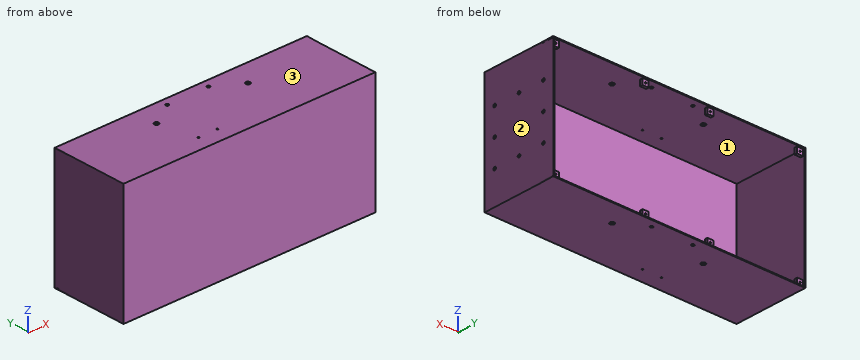
from build123d import *

# Parameters (mm, degrees)
SKETCH1_W            = 855
SKETCH1_H            = 400
BOSS_EXTRUDE1_DEPTH  = 4
SKETCH3_W            = 3
SKETCH3_H            = 394
BOSS_EXTRUDE2_DEPTH  = 200
BOSS_EXTRUDE3_DEPTH  = 3
BOSS_EXTRUDE4_START  = -3
BOSS_EXTRUDE4_DEPTH  = 3
SKETCH10_R           = 5
CUT_EXTRUDE4_DEPTH   = 639.178854241
SKETCH11_R           = 2.5
CUT_EXTRUDE5_DEPTH   = 639.178854241
BOSS_EXTRUDE7_DEPTH  = 3
BOSS_EXTRUDE10_START = -3
BOSS_EXTRUDE10_DEPTH = 3
SKETCH33_W           = 3
SKETCH33_H           = 394
BOSS_EXTRUDE14_DEPTH = 50
SKETCH34_W           = 3
SKETCH34_H           = 394
BOSS_EXTRUDE15_DEPTH = 50
SKETCH36_W           = 20
SKETCH36_H           = 20
BOSS_EXTRUDE16_DEPTH = 9
SKETCH40_R           = 2.5
CUT_EXTRUDE6_DEPTH   = 9
SKETCH44_W           = 20
SKETCH44_H           = 20
BOSS_EXTRUDE18_DEPTH = 9
SKETCH45_R           = 2.5
CUT_EXTRUDE7_DEPTH   = 9
SKETCH46_W           = 20
SKETCH46_H           = 20
BOSS_EXTRUDE19_DEPTH = 9
SKETCH47_R           = 2.5
CUT_EXTRUDE8_DEPTH   = 9
SKETCH48_W           = 20
SKETCH48_H           = 20
BOSS_EXTRUDE20_DEPTH = 9
SKETCH49_R           = 2.5
CUT_EXTRUDE9_DEPTH   = 9
SKETCH50_W           = 20
SKETCH50_H           = 20
BOSS_EXTRUDE21_DEPTH = 9
SKETCH51_R           = 2.5
CUT_EXTRUDE10_DEPTH  = 9
SKETCH52_W           = 20
SKETCH52_H           = 20
BOSS_EXTRUDE22_DEPTH = 9
SKETCH53_R           = 2.5
CUT_EXTRUDE11_DEPTH  = 9
SKETCH58_W           = 20
SKETCH58_H           = 20
BOSS_EXTRUDE25_DEPTH = 9
SKETCH61_R           = 2.5
CUT_EXTRUDE13_DEPTH  = 9
SKETCH62_W           = 20
SKETCH62_H           = 20
BOSS_EXTRUDE26_DEPTH = 9
SKETCH63_R           = 2.5
CUT_EXTRUDE14_DEPTH  = 9
SKETCH64_R           = 7.5
CUT_EXTRUDE15_DEPTH  = 639.906527631
SKETCH65_R           = 5
CUT_EXTRUDE16_DEPTH  = 3


with BuildPart() as part:
    # Sketch1 → Boss-Extrude1 (new body)
    with BuildSketch(Plane(origin=(0, 0, 0), x_dir=(1, 0, 0), z_dir=(0, 1, 0))):
        Rectangle(SKETCH1_W, SKETCH1_H)
    extrude(amount=BOSS_EXTRUDE1_DEPTH)

    # Sketch3 → Boss-Extrude2 (add)
    with BuildSketch(Plane(origin=(0, 4, 0), x_dir=(1, 0, 0), z_dir=(0, 1, 0))):
        Polygon((-424.5, 200), (-424.5, 197), (424.5, 197), (427.5, 197), (427.5, 200), align=None)
        with Locations((426, 0)):
            Rectangle(SKETCH3_W, SKETCH3_H)
        Polygon((-427.5, -197), (-427.5, -200), (427.5, -200), (427.5, -197), (424.5, -197), (-424.5, -197), align=None)
        Polygon((-427.5, 200), (-427.5, -197), (-424.5, -197), (-424.5, 197), (-424.5, 200), align=None)
    extrude(amount=BOSS_EXTRUDE2_DEPTH)

    # Sketch4 → Boss-Extrude3 (add)
    with BuildSketch(Plane.XY.offset(200)):
        with BuildLine():
            ThreePointArc((427.5, 204), (215.207022423, 241.457541713), (0, 254))
            Line((0, 254), (0, 204))
            Line((0, 204), (427.5, 204))
        make_face()
        with BuildLine():
            Line((0, 204), (0, 254))
            ThreePointArc((0, 254), (-215.207022423, 241.457541713), (-427.5, 204))
            Line((-427.5, 204), (0, 204))
        make_face()
        with BuildLine():
            ThreePointArc((427.5, 204), (215.207022423, 241.457541713), (0, 254))
            Line((0, 254), (0, 204))
            Line((0, 204), (427.5, 204))
        make_face()
        with BuildLine():
            Line((0, 204), (0, 254))
            ThreePointArc((0, 254), (-215.207022423, 241.457541713), (-427.5, 204))
            Line((-427.5, 204), (0, 204))
        make_face()
    extrude(amount=-BOSS_EXTRUDE3_DEPTH)

    # Sketch6 → Boss-Extrude4 (add)
    with BuildSketch(Plane(origin=(0, 0, -200), x_dir=(-1, 0, 0), z_dir=(0, 0, -1)).offset(BOSS_EXTRUDE4_START)):
        with BuildLine():
            ThreePointArc((427.5, 204), (215.207022423, 241.457541713), (0, 254))
            Line((0, 254), (0, 204))
            Line((0, 204), (427.5, 204))
        make_face()
        with BuildLine():
            Line((0, 204), (0, 254))
            ThreePointArc((0, 254), (-215.207022423, 241.457541713), (-427.5, 204))
            Line((-427.5, 204), (0, 204))
        make_face()
        with BuildLine():
            ThreePointArc((427.5, 204), (215.207022423, 241.457541713), (0, 254))
            Line((0, 254), (0, 204))
            Line((0, 204), (427.5, 204))
        make_face()
        with BuildLine():
            Line((0, 204), (0, 254))
            ThreePointArc((0, 254), (-215.207022423, 241.457541713), (-427.5, 204))
            Line((-427.5, 204), (0, 204))
        make_face()
    extrude(amount=BOSS_EXTRUDE4_DEPTH)

    # Sketch10 → Cut-Extrude4 (cut, through all)
    with BuildSketch(Plane.XY.offset(200)):
        with Locations((70, 227.5)):
            Circle(SKETCH10_R)
        with Locations((-70, 227.5)):
            Circle(SKETCH10_R)
    extrude(amount=-CUT_EXTRUDE4_DEPTH, mode=Mode.SUBTRACT)

    # Sketch11 → Cut-Extrude5 (cut, through all)
    with BuildSketch(Plane.XY.offset(200)):
        with Locations((-63, 50)):
            Circle(SKETCH11_R)
        with Locations((-127, 50)):
            Circle(SKETCH11_R)
    extrude(amount=-CUT_EXTRUDE5_DEPTH, mode=Mode.SUBTRACT)

    # Sketch12 → Boss-Extrude7 (add)
    with BuildSketch(Plane.XY.offset(200)):
        with BuildLine():
            Line((428.585523611, 254), (0, 254))
            ThreePointArc((0, 254), (215.207022423, 241.457541713), (427.5, 204))
            Line((427.5, 204), (428.585523611, 254))
        make_face()
        with BuildLine():
            ThreePointArc((-427.5, 204), (-215.207022423, 241.457541713), (0, 254))
            Line((0, 254), (-427.66164317, 254))
            Line((-427.66164317, 254), (-427.5, 204))
        make_face()
    extrude(amount=-BOSS_EXTRUDE7_DEPTH)

    # Sketch23 → Boss-Extrude10 (add)
    # profile 1 of 2: a face of its own
    with BuildSketch(Plane(origin=(0, 0, -200), x_dir=(-1, 0, 0), z_dir=(0, 0, -1)).offset(BOSS_EXTRUDE10_START)):
        with BuildLine():
            Line((-428.585523611, 254), (-427.5, 204))
            add(Edge.make_bspline(
                [(-427.5, 204), (-213.75, 254), (0, 254)],
                knots=[0, 0, 0, 0.5, 0.5, 0.5], degree=2))
            Line((0, 254), (-428.585523611, 254))
        make_face()
    # profile 2 of 2: a face of its own
    with BuildSketch(Plane(origin=(0, 0, -200), x_dir=(-1, 0, 0), z_dir=(0, 0, -1)).offset(BOSS_EXTRUDE10_START)):
        with BuildLine():
            Line((427.66164317, 254), (0, 254))
            add(Edge.make_bspline(
                [(0, 254), (213.75, 254), (427.5, 204)],
                knots=[0.5, 0.5, 0.5, 1, 1, 1], degree=2))
            Line((427.5, 204), (427.66164317, 254))
        make_face()
        with BuildLine():
            ThreePointArc((0, 254), (215.207022423, 241.457541713), (427.5, 204))
            add(Edge.make_bspline(
                [(0, 254), (213.75, 254), (427.5, 204)],
                knots=[0.5, 0.5, 0.5, 1, 1, 1], degree=2))
        make_face(mode=Mode.SUBTRACT)
    extrude(amount=BOSS_EXTRUDE10_DEPTH)

    # Sketch33 → Boss-Extrude14 (add)
    with BuildSketch(Plane(origin=(0, 204, 0), x_dir=(1, 0, 0), z_dir=(0, 1, 0))):
        with Locations((-426, 0)):
            Rectangle(SKETCH33_W, SKETCH33_H)
    extrude(amount=BOSS_EXTRUDE14_DEPTH)

    # Sketch34 → Boss-Extrude15 (add)
    with BuildSketch(Plane(origin=(0, 204, 0), x_dir=(1, 0, 0), z_dir=(0, 1, 0))):
        with Locations((426, 0)):
            Rectangle(SKETCH34_W, SKETCH34_H)
    extrude(amount=BOSS_EXTRUDE15_DEPTH)

    # Sketch36 → Boss-Extrude16 (add)
    with BuildSketch(Plane(origin=(0, 240, 0), x_dir=(1, 0, 0), z_dir=(0, 1, 0))):
        with Locations((-414.5, 187)):
            Rectangle(SKETCH36_W, SKETCH36_H)
    extrude(amount=BOSS_EXTRUDE16_DEPTH)

    # Sketch40 → Cut-Extrude6 (cut)
    with BuildSketch(Plane(origin=(0, 254, 0), x_dir=(1, 0, 0), z_dir=(0, 1, 0))):
        with Locations(Location((-414.5, 187, 0), (0, 0, 270))):
            Circle(SKETCH40_R)
    extrude(amount=-CUT_EXTRUDE6_DEPTH, mode=Mode.SUBTRACT)

    # Sketch44 → Boss-Extrude18 (add)
    with BuildSketch(Plane(origin=(0, 240, 0), x_dir=(1, 0, 0), z_dir=(0, 1, 0))):
        with Locations((-414.5, -187)):
            Rectangle(SKETCH44_W, SKETCH44_H)
    extrude(amount=BOSS_EXTRUDE18_DEPTH)

    # Sketch45 → Cut-Extrude7 (cut)
    with BuildSketch(Plane(origin=(0, 254, 0), x_dir=(1, 0, 0), z_dir=(0, 1, 0))):
        with Locations(Location((-414.5, -187, 0), (0, 0, 270))):
            Circle(SKETCH45_R)
    extrude(amount=-CUT_EXTRUDE7_DEPTH, mode=Mode.SUBTRACT)

    # Sketch46 → Boss-Extrude19 (add)
    with BuildSketch(Plane(origin=(0, 240, 0), x_dir=(1, 0, 0), z_dir=(0, 1, 0))):
        with Locations((414.5, 187)):
            Rectangle(SKETCH46_W, SKETCH46_H)
    extrude(amount=BOSS_EXTRUDE19_DEPTH)

    # Sketch47 → Cut-Extrude8 (cut)
    with BuildSketch(Plane(origin=(0, 254, 0), x_dir=(1, 0, 0), z_dir=(0, 1, 0))):
        with Locations(Location((414.5, 187, 0), (0, 0, 270))):
            Circle(SKETCH47_R)
    extrude(amount=-CUT_EXTRUDE8_DEPTH, mode=Mode.SUBTRACT)

    # Sketch48 → Boss-Extrude20 (add)
    with BuildSketch(Plane(origin=(0, 240, 0), x_dir=(1, 0, 0), z_dir=(0, 1, 0))):
        with Locations((414.5, -187)):
            Rectangle(SKETCH48_W, SKETCH48_H)
    extrude(amount=BOSS_EXTRUDE20_DEPTH)

    # Sketch49 → Cut-Extrude9 (cut)
    with BuildSketch(Plane(origin=(0, 254, 0), x_dir=(1, 0, 0), z_dir=(0, 1, 0))):
        with Locations(Location((414.5, -187, 0), (0, 0, 270))):
            Circle(SKETCH49_R)
    extrude(amount=-CUT_EXTRUDE9_DEPTH, mode=Mode.SUBTRACT)

    # Sketch50 → Boss-Extrude21 (add)
    with BuildSketch(Plane(origin=(0, 240, 0), x_dir=(1, 0, 0), z_dir=(0, 1, 0))):
        with Locations((110, 187)):
            Rectangle(SKETCH50_W, SKETCH50_H)
    extrude(amount=BOSS_EXTRUDE21_DEPTH)

    # Sketch51 → Cut-Extrude10 (cut)
    with BuildSketch(Plane(origin=(0, 254, 0), x_dir=(1, 0, 0), z_dir=(0, 1, 0))):
        with Locations(Location((110, 187, 0), (0, 0, 270))):
            Circle(SKETCH51_R)
    extrude(amount=-CUT_EXTRUDE10_DEPTH, mode=Mode.SUBTRACT)

    # Sketch52 → Boss-Extrude22 (add)
    with BuildSketch(Plane(origin=(0, 240, 0), x_dir=(1, 0, 0), z_dir=(0, 1, 0))):
        with Locations((110, -187)):
            Rectangle(SKETCH52_W, SKETCH52_H)
    extrude(amount=BOSS_EXTRUDE22_DEPTH)

    # Sketch53 → Cut-Extrude11 (cut)
    with BuildSketch(Plane(origin=(0, 254, 0), x_dir=(1, 0, 0), z_dir=(0, 1, 0))):
        with Locations(Location((110, -187, 0), (0, 0, 270))):
            Circle(SKETCH53_R)
    extrude(amount=-CUT_EXTRUDE11_DEPTH, mode=Mode.SUBTRACT)

    # Sketch58 → Boss-Extrude25 (add)
    with BuildSketch(Plane(origin=(0, 240, 0), x_dir=(1, 0, 0), z_dir=(0, 1, 0))):
        with Locations((-110, 187)):
            Rectangle(SKETCH58_W, SKETCH58_H)
    extrude(amount=BOSS_EXTRUDE25_DEPTH)

    # Sketch61 → Cut-Extrude13 (cut)
    with BuildSketch(Plane(origin=(0, 254, 0), x_dir=(1, 0, 0), z_dir=(0, 1, 0))):
        with Locations(Location((-110, 187, 0), (0, 0, 270))):
            Circle(SKETCH61_R)
    extrude(amount=-CUT_EXTRUDE13_DEPTH, mode=Mode.SUBTRACT)

    # Sketch62 → Boss-Extrude26 (add)
    with BuildSketch(Plane(origin=(0, 240, 0), x_dir=(1, 0, 0), z_dir=(0, 1, 0))):
        with Locations((-110, -187)):
            Rectangle(SKETCH62_W, SKETCH62_H)
    extrude(amount=BOSS_EXTRUDE26_DEPTH)

    # Sketch63 → Cut-Extrude14 (cut)
    with BuildSketch(Plane(origin=(0, 254, 0), x_dir=(1, 0, 0), z_dir=(0, 1, 0))):
        with Locations(Location((-110, -187, 0), (0, 0, 270))):
            Circle(SKETCH63_R)
    extrude(amount=-CUT_EXTRUDE14_DEPTH, mode=Mode.SUBTRACT)

    # Sketch64 → Cut-Extrude15 (cut, through all)
    with BuildSketch(Plane.XY.offset(200)):
        with Locations((155, 174)):
            Circle(SKETCH64_R)
        with Locations((-155, 174)):
            Circle(SKETCH64_R)
    extrude(amount=-CUT_EXTRUDE15_DEPTH, mode=Mode.SUBTRACT)

    # Sketch65 → Cut-Extrude16 (cut)
    with BuildSketch(Plane(origin=(427.5, 0, 0), x_dir=(0, 0, -1), z_dir=(1, 0, 0))):
        with Locations((90, 216.999992336)):
            Circle(SKETCH65_R)
        with Locations((0, 216.999996168)):
            Circle(SKETCH65_R)
        with Locations((-90, 217)):
            Circle(SKETCH65_R)
        with Locations((-90, 127)):
            Circle(SKETCH65_R)
        with Locations((90, 127)):
            Circle(SKETCH65_R)
        with Locations((90, 36.999996168)):
            Circle(SKETCH65_R)
        with Locations((0, 36.999996168)):
            Circle(SKETCH65_R)
        with Locations((-90, 37)):
            Circle(SKETCH65_R)
    extrude(amount=-CUT_EXTRUDE16_DEPTH, mode=Mode.SUBTRACT)


solid = part.part
Work out the finished part from the listing and answer in its coordinate system (mm). Face numbers are marked on the shaded views. Give positions to 0.01 mm unless a question says otherwise; leave off trailing zeros. Order: outer loops, then holes, each group sorted by start corner. A loop starts at its lowest first (then second) coordinate and runs counter-clockwise, first axis right, second up. Notation, with made-up numbers: (42, 81.5) -> (70, 81.5) arc R16 ccw to (70, 89.5) -> close; hole circle Ø3 at (36.5, -36). An arc over 180 degrees is marked (long way). Answer as a JSON object with one key per item and string values. Group by question number.
1. Section A-A on y = 102 is taken. Determine the outline of the cut face in (x, z).
2. Consider line 1 along Y through (x, z) = (426.9, -90); line 2 along Z through (x, y) = (-210, 99); line 3 along X through (y, z) = (183, 51). Determine where each line is inside the solid, lowest interval first. Write a range as [from, to].
3. The mould has two halves that part along X. Classify the marked faces 1, 2 and 3: released by +X, released by -X, zero draft, split by the parting line, or undercut.
4. Section C-C on x = 312 is taken. Determine the outline of the cut face in (y, z).
5. Flat-ended cylindrical pins translate along their axes: pin 1 Ø10 at (y, z) = (155.5, 142) entering from +X; pin 2 Ø1 at (y, z) = (66.5, -125.5) entering from -X; pin 3 Ø6 at (x, z) = (417, -190) entering from +Y. Find the tip coordinate at first contact, or state that the pin passes through.
6. Section B-B on z = 64.5 is taken. Determine the outline of the cut face in (x, y), plus the area to 3 significant figures.
Result sheet:
{
 "1": {"outline": "(-427.5, -200) -> (427.5, -200) -> (427.5, 200) -> (-427.5, 200) -> close; hole (-424.5, -197) -> (424.5, -197) -> (424.5, 197) -> (-424.5, 197) -> close"},
 "2": {"line 1": "y = [0, 32], [42, 122], [132, 212], [222, 254]", "line 2": "z = [-200, -197], [197, 200]", "line 3": "x = [-427.5, -424.5], [424.5, 427.5]"},
 "3": {"face 1": "undercut", "face 2": "released by +X", "face 3": "zero draft"},
 "4": {"outline": "(0, -200) -> (254, -200) -> (254, -197) -> (4, -197) -> (4, 197) -> (254, 197) -> (254, 200) -> (0, 200) -> close"},
 "5": {"pin 1": "stops at x = 427.5", "pin 2": "stops at x = -427.5", "pin 3": "stops at y = 249"},
 "6": {"outline": "(-427.5, 0) -> (427.5, 0) -> (427.5, 254) -> (424.5, 254) -> (424.5, 4) -> (-424.5, 4) -> (-424.5, 254) -> (-427.5, 254) -> close", "area": "4,920 mm^2"}
}
